```python
from build123d import *

# Parameters (mm, degrees)
F0_R     = 1.25
F1_DEPTH = 1.6
F2_W     = 2.54
F2_H     = 25.4
F3_DEPTH = 1.27
F4_W     = 5.605
F4_H     = 18
F5_DEPTH = 1.27


with BuildPart() as f1:
    # F0 (on Top) → F1 (new body)
    with BuildSketch(Plane.XY):
        with BuildLine():
            Line((12.065, 17.78), (-12.065, 17.78))
            ThreePointArc((-12.065, 17.78), (-13.861051, 17.036051), (-14.605, 15.24))
            Line((-14.605, 15.24), (-14.605, -15.24))
            ThreePointArc((-14.605, -15.24), (-13.861051, -17.036051), (-12.065, -17.78))
            Line((-12.065, -17.78), (12.065, -17.78))
            ThreePointArc((12.065, -17.78), (13.861051, -17.036051), (14.605, -15.24))
            Line((14.605, -15.24), (14.605, 15.24))
            ThreePointArc((14.605, 15.24), (13.861051, 17.036051), (12.065, 17.78))
        make_face()
        with Locations((-12.065, -15.24)):
            Circle(F0_R, mode=Mode.SUBTRACT)
        with Locations((12.065, -15.24)):
            Circle(F0_R, mode=Mode.SUBTRACT)
        with Locations((-12.065, 15.24)):
            Circle(F0_R, mode=Mode.SUBTRACT)
        with Locations((12.065, 15.24)):
            Circle(F0_R, mode=Mode.SUBTRACT)
    extrude(amount=-F1_DEPTH)

    # F2 (on Top) → F3 (join)
    with BuildSketch(Plane.XY):
        with Locations((-12.065, 0)):
            Rectangle(F2_W, F2_H)
    extrude(amount=F3_DEPTH)

    # F4 (on face) → F5 (join)
    with BuildSketch(Plane.XY):
        Polygon((-9, -12), (9, -12), (9, -9), (9, 9), (9, 12), (-9, 12), align=None)
        with Locations((11.8025, 0)):
            Rectangle(F4_W, F4_H)
    extrude(amount=F5_DEPTH)


solid = f1.part
```
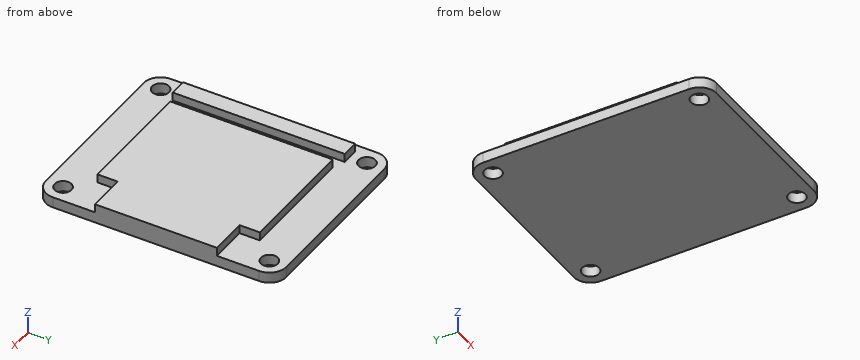
The listing builds one solid part. Answer for the finished solid, in the listing's coordinates (mm). Round coordinates to 2 decimals unless told otherwise and drop trailing zeros. Loops run counter-clockwise (first coordinate to the right, second up) from the corner with the lowest first, then second, coordinate; pieces in that order, holes last.
Q1. Section B-B, the plane y = -8.5 is taken. Determine the outline of the cut face in (x, z) (3 decimals), then the cut area to 3 significant figures.
Q2. Section D-D, the plane y = 16 is taken. Determine the outline of the cut face in (x, z), then the cut area to 3 significant figures.
Q3. Section A-A, the plane z = 0.85 is taken. Determine the outline of the cut face in (x, y) (3 decimals), then the cut area to 3 significant figures.
Q4. Section C-C, the plane x = -3.5 is taken. Determine the outline of the cut face in (y, z).
Q5. Given pin 1 Ø1 at (y, z) = (-2.5, 1) entering from -X (3 decimals); pin 2 Ø1.4 at (x, z) = (13, 0.5) entering from -Y; pin 3 Ø1 at (y, z) = (-10, 1) entering from +X, each flat-ended and moving along its own axis, determine where each tip first touches the part or whether it passes through.
Q6. Find the intervals of material crossed by line 1 (X direction, y = 14.5, z = -0.55) (3 decimals); line 2 (X direction, y = -8, z = 0.8) (3 decimals); line 3 (X direction, y = -11, z = 1.1) (3 decimals), in increasing order.
Completed:
1. outline: (-14.605, -1.6) - (14.605, -1.6) - (14.605, 1.27) - (-9, 1.27) - (-9, 0) - (-10.795, 0) - (-10.795, 1.27) - (-13.335, 1.27) - (-13.335, 0) - (-14.605, 0) - close
1. area: 79.9 mm2
2. outline: (-14.49, -1.6) - (-13.06, -1.6) - (-13.06, 0) - (-14.49, 0) - close; (-11.07, -1.6) - (11.07, -1.6) - (11.07, 0) - (-11.07, 0) - close; (13.06, -1.6) - (14.49, -1.6) - (14.49, 0) - (13.06, 0) - close
2. area: 40.0 mm2
3. outline: (-13.335, -12.7) - (-10.795, -12.7) - (-10.795, 12.7) - (-13.335, 12.7) - close; (-9, -12) - (9, -12) - (9, -9) - (14.605, -9) - (14.605, 9) - (9, 9) - (9, 12) - (-9, 12) - close
3. area: 597 mm2
4. outline: (-17.78, -1.6) - (17.78, -1.6) - (17.78, 0) - (12, 0) - (12, 1.27) - (-12, 1.27) - (-12, 0) - (-17.78, 0) - close
5. pin 1: stops at x = -13.335
5. pin 2: stops at y = -17.74
5. pin 3: stops at x = 9
6. line 1: x = -14.605 to -13.072, -11.058 to 11.058, 13.072 to 14.605
6. line 2: x = -13.335 to -10.795, -9 to 14.605
6. line 3: x = -13.335 to -10.795, -9 to 9
